For this review, take the finished solid that the model builds, in its own axes (mm). Face numbers are marked on the shaded views. Coordinates: 2 decimals unless noted, no trailing zeros. Loops run counter-clockwise (first coordinate to the right, second up) from the corner with the lowest first, then second, coordinate; pieces in that order, holes last. Notation, with made-up numbers: (59.25, 23) - (101.25, 23) arc R5 ccw to (101.25, 30) - close; hole circle Ø4 at (78.25, 2.5). An arc over 180 degrees is marked (long way). Answer as a JSON object with one key per item and string values. Group by question number.
Item 1: To check wall thickness, follow line 1 (X direction, y = -3.5, z = 1.75); line 2 (Z direction, x = -1.5, y = 0.25); line 3 (Z direction, x = 3.75, y = -0.5). State the ranges of each line that lie inside material, in increasing order.
Item 2: Clearance check with flat-ended pins moving along their axes: pin 1 (3.5 mm diameter, centred on x = 2.5, y = -3, fed in from -Z); pin 2 (0.8 mm diameter, centred on x = 3.5, z = -2.5, fed in from +Y); pin 3 (0.5 mm diameter, centred on y = 4.5, z = -1, fed in from +X). State where each tip first meets the part, or that it passes through.
Item 3: Mouldability with a two-part tool opening along Z and no side actions: class the marked faces 1, 2, 3 and 4 as released by +Z, released by -Z, zero draft, split by the parting line, or undercut.
Item 4: We need section A-A (x = 3.5). Give the boundary of the cut face in (y, z).
Item 5: We need section C-C (y = 1.5). Give the boundary of the cut face in (x, z), then the cut area to 3 significant figures.
Item 6: We need section D-D (x = 1). Give the boundary of the cut face in (y, z), then the cut area to 3 significant figures.
Item 7: We need section B-B (z = 5). Give the boundary of the cut face in (x, y).
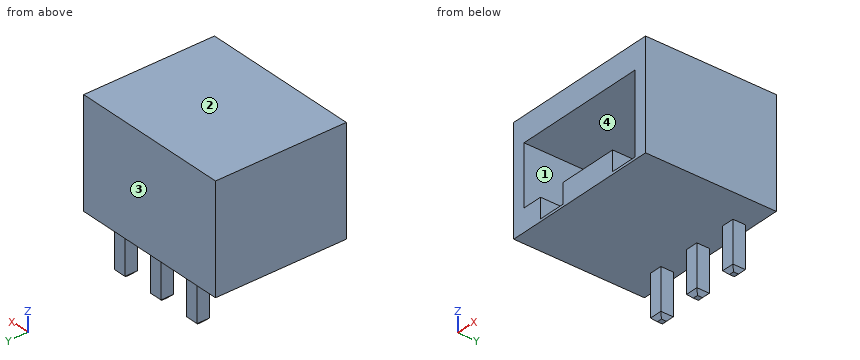
from build123d import *

# Parameters (mm, degrees)
SKETCH_1_W                         = 12.8
SKETCH_1_H                         = 10.5
EXTRUDE_1_DEPTH                    = 8.6
CUT_EXTRUDE_1_DEPTH                = 7
EXTRUDE_START                      = -5
SKETCH_3_W                         = 1
SKETCH_3_H                         = 1
EXTRUDE_2_DEPTH                    = 8.6
CHAMFER_1_SIZE                     = 0.3
PATTERN_LINEAR_1_COUNT             = 3
PATTERN_LINEAR_1_PITCH             = 3.5
CHAMFER_1_OF_PATTERN_LINEAR_1_SIZE = 0.3


with BuildPart() as part:
    # Эскиз1 → Бобышка-Вытянуть1 (new body)
    with BuildSketch(Plane.XY):
        Rectangle(SKETCH_1_W, SKETCH_1_H)
    extrude(amount=EXTRUDE_1_DEPTH)

    # Эскиз2 → Вырез-Вытянуть1 (cut)
    with BuildSketch(Plane.XZ.offset(5.25)):
        Polygon((-5.4, 6.6), (5.4, 6.6), (5.4, 0.2), (3.2, 0.2), (3.2, 1.8), (-1.6, 1.8), (-1.6, 0.2), (-3.8, 0.2), (-3.8, 1.8), (-5.4, 1.8), align=None)
    extrude(amount=-CUT_EXTRUDE_1_DEPTH, mode=Mode.SUBTRACT)

    # Эскиз3 → Бобышка-Вытянуть2 (add)
    with BuildSketch(Plane(origin=(0, 0, 0), x_dir=(-1, 0, 0), z_dir=(0, 0, -1)).offset(EXTRUDE_START)):
        with Locations((3.5, 4.25)):
            Rectangle(SKETCH_3_W, SKETCH_3_H)
    extrude_2 = extrude(amount=EXTRUDE_2_DEPTH)

    # Фаска1
    chamfer_1_edges = [part.edges().sort_by_distance(p)[0] for p in [
        (-3, 4.25, -3.6),
        (-3.5, 3.75, -3.6),
        (-4, 4.25, -3.6),
        (-3.5, 4.75, -3.6),
    ]]
    chamfer(chamfer_1_edges, length=CHAMFER_1_SIZE)

    # Линейный массив1: Бобышка-Вытянуть2 ×3
    with Locations(*[(i * PATTERN_LINEAR_1_PITCH, 0, 0) for i in range(1, PATTERN_LINEAR_1_COUNT)]):
        add(extrude_2)

    # Фаска1 of Линейный массив1
    chamfer_1_of_pattern_linear_1_edges = [part.edges().sort_by_distance(p)[0] for p in [
        (0.5, 4.25, -3.6),
        (0, 3.75, -3.6),
        (-0.5, 4.25, -3.6),
        (0, 4.75, -3.6),
        (4, 4.25, -3.6),
        (3.5, 3.75, -3.6),
        (3, 4.25, -3.6),
        (3.5, 4.75, -3.6),
    ]]
    chamfer(chamfer_1_of_pattern_linear_1_edges, length=CHAMFER_1_OF_PATTERN_LINEAR_1_SIZE)


solid = part.part
Check sheet entries:
{
 "1": {"line 1": "x = -6.4 to -3.8, -1.6 to 3.2, 5.4 to 6.4", "line 2": "z = 0 to 1.8, 6.6 to 8.6", "line 3": "z = 0 to 0.2, 6.6 to 8.6"},
 "2": {"pin 1": "stops at z = 0", "pin 2": "stops at y = 4.75", "pin 3": "stops at x = 4"},
 "3": {"face 1": "undercut", "face 2": "released by +Z", "face 3": "zero draft", "face 4": "undercut"},
 "4": {"outline": "(-5.25, 0) - (3.75, 0) - (3.75, -3.3) - (4.05, -3.6) - (4.45, -3.6) - (4.75, -3.3) - (4.75, 0) - (5.25, 0) - (5.25, 8.6) - (-5.25, 8.6) - (-5.25, 6.6) - (1.75, 6.6) - (1.75, 0.2) - (-5.25, 0.2) - close"},
 "5": {"outline": "(-6.4, 0) - (6.4, 0) - (6.4, 8.6) - (-6.4, 8.6) - close; hole (-5.4, 1.8) - (-3.8, 1.8) - (-3.8, 0.2) - (-1.6, 0.2) - (-1.6, 1.8) - (3.2, 1.8) - (3.2, 0.2) - (5.4, 0.2) - (5.4, 6.6) - (-5.4, 6.6) - close", "area": "51.2 mm2"},
 "6": {"outline": "(-5.25, 0) - (5.25, 0) - (5.25, 8.6) - (-5.25, 8.6) - (-5.25, 6.6) - (1.75, 6.6) - (1.75, 1.8) - (-5.25, 1.8) - close", "area": "56.7 mm2"},
 "7": {"outline": "(-6.4, -5.25) - (-5.4, -5.25) - (-5.4, 1.75) - (5.4, 1.75) - (5.4, -5.25) - (6.4, -5.25) - (6.4, 5.25) - (-6.4, 5.25) - close"}
}
